from build123d import *

# Parameters (mm, degrees)
F0_W     = 140
F0_H     = 140
F0_R     = 50
F1_DEPTH = 17.5
F2_W     = 10
F2_H     = 140
F3_DEPTH = 15
F5_DEPTH = 18
F7_DEPTH = 172.6


with BuildPart() as f1:
    # F0 (on Top) → F1 (new body, symmetric)
    with BuildSketch(Plane.XY):
        Rectangle(F0_W, F0_H)
        with Locations((0, 3.96405)):
            Circle(F0_R, mode=Mode.SUBTRACT)
    extrude(amount=F1_DEPTH, both=True)

    # F2 (on face) → F3 (cut)
    with BuildSketch(Plane.XY.offset(17.5)):
        with Locations((-60, 0)):
            Rectangle(F2_W, F2_H)
    extrude(amount=-F3_DEPTH, mode=Mode.SUBTRACT)

    # F4 (on face) → F5 (cut)
    with BuildSketch(Plane.XY.offset(17.5)):
        with BuildLine():
            Line((22.5, -70), (22.5, -40.687378))
            ThreePointArc((22.5, -40.687378), (0, -46.03595), (-22.5, -40.687378))
            Line((-22.5, -40.687378), (-22.5, -70))
            Line((-22.5, -70), (22.5, -70))
        make_face()
        with BuildLine():
            Line((22.5, 48.615477), (22.5, 70))
            Line((22.5, 70), (-22.5, 70))
            Line((-22.5, 70), (-22.5, 48.615477))
            ThreePointArc((-22.5, 48.615477), (0, 53.96405), (22.5, 48.615477))
        make_face()
    extrude(amount=-F5_DEPTH, mode=Mode.SUBTRACT)

    # F6 (on face) → F7 (cut)
    with BuildSketch(Plane.XZ.offset(70)):
        Polygon((52.595693, 17.5), (42.595693, 17.5), (32.203389, -0.5), (62.987998, -0.5), align=None)
    extrude(amount=-F7_DEPTH, mode=Mode.SUBTRACT)


solid = f1.part
Geometry check sheet. Reference: the model listing, model coordinates, mm. A direction names the side the tool comes from. Round coordinates to 2 decimals unless told otherwise and drop trailing zeros. Loops run counter-clockwise (first coordinate to the right, second up) from the corner with the lowest first, then second, coordinate; pieces in that order, holes last. Notation, with made-up numbers: (56.25, -15) -> (112.25, -15) arc R4 ccw to (112.25, -11) -> close; hole circle Ø2 at (-4.75, 28). An arc over 180 degrees is marked (long way). Answer as a JSON object with one key per item and string values. Group by question number.
Item 1: Depth check by flat-ended pin: pin 1 Ø5 at (x, y) = (-62, -2.5) entering from +Z; pin 2 Ø10.5 at (x, y) = (6, 62) entering from +Z. Enter the tip coordinate at first touch or a pass-through.
Item 2: Thickness scan on line 1 along X through (y, z) = (21, 10.5); line 2 along X through (y, z) = (-16, 11.5); line 3 along Y through (x, z) = (0, -10). Record the ranges inside material, lowest first.
Item 3: Cross-section at B-B, the plane y = 35. Record the cut outline in (x, z).
Item 4: Release check for a two-part mould opening along Z. For faces 3 (the face through (51, -1, -0.5)), 4 (the face through (32, -51, 17.5)), 5 (the face through (-1, -70, -4)) record: pulls with the +Z half, pulls with the -Z half, needs draft (parallel to the pull), parting line crosses it, or undercut.
Item 5: Cross-section at A-A, the plane x = 0. Record the cut outline in (y, z).
Item 6: Cross-section at C-C, the plane z = 9.5. Record the cut outline in (x, y), plus the area to 3 significant figures.
Item 7: Set-up check for faces 1 (the face through (22.5, 59, 9)), 2 (the face through (-53, 1, 17.5)): record each of +Z, -Z, +X, -X, +Y, -Y from which the full face is reachable in a straight line by a thin tool's end or side.
Item 8: Cross-section at D-D, the plane x = 37. Record the cut outline in (y, z), plus the area to 3 significant figures.
Determined:
{
 "1": {"pin 1": "stops at z = 2.5", "pin 2": "stops at z = -0.5"},
 "2": {"line 1": "x = -70 to -65, -55 to -47.01, 56.64 to 70", "line 2": "x = -70 to -65, -55 to -45.84, 56.06 to 70", "line 3": "y = -70 to -46.04, 53.96 to 70"},
 "3": {"outline": "(-70, -17.5) -> (-39.2, -17.5) -> (-39.2, 17.5) -> (-55, 17.5) -> (-55, 2.5) -> (-65, 2.5) -> (-65, 17.5) -> (-70, 17.5) -> close; (39.2, -17.5) -> (70, -17.5) -> (70, 17.5) -> (52.6, 17.5) -> (62.99, -0.5) -> (39.2, -0.5) -> close; (39.2, 11.62) -> (42.6, 17.5) -> (39.2, 17.5) -> close"},
 "4": {"face 3": "undercut", "face 4": "pulls with the +Z half", "face 5": "needs draft"},
 "5": {"outline": "(-70, -17.5) -> (-46.04, -17.5) -> (-46.04, -0.5) -> (-70, -0.5) -> close; (53.96, -17.5) -> (70, -17.5) -> (70, -0.5) -> (53.96, -0.5) -> close"},
 "6": {"outline": "(-70, -70) -> (-65, -70) -> (-65, 70) -> (-70, 70) -> close; (-55, -70) -> (-22.5, -70) -> (-22.5, -40.69) arc R50 cw to (-22.5, 48.62) -> (-22.5, 70) -> (-55, 70) -> close; (22.5, -70) -> (37.98, -70) -> (37.98, -28.56) arc R50 cw to (22.5, -40.69) -> close; (22.5, 48.62) arc R50 cw to (37.98, 36.49) -> (37.98, 70) -> (22.5, 70) -> close; (57.21, -70) -> (70, -70) -> (70, 70) -> (57.21, 70) -> close", "area": "6,230 mm²"},
 "7": {"face 1": "+Z, +Y, -Y", "face 2": "+Z, +X, -X, +Y, -Y"},
 "8": {"outline": "(-70, -17.5) -> (-29.67, -17.5) -> (-29.67, -0.5) -> (-70, -0.5) -> close; (-70, 7.81) -> (-29.67, 7.81) -> (-29.67, 17.5) -> (-70, 17.5) -> close; (37.59, -17.5) -> (70, -17.5) -> (70, -0.5) -> (37.59, -0.5) -> close; (37.59, 7.81) -> (70, 7.81) -> (70, 17.5) -> (37.59, 17.5) -> close", "area": "1,940 mm²"}
}
